Geometry check sheet. Reference: the model listing, model coordinates, mm. Face numbers are marked on the shaded views. A direction names the side the tool comes from. Give positions to 0.01 mm unless a question says otherwise; leave off trailing zeros. Write each loop counter-clockwise with the first axis right and the second up, starting at its lowest first coordinate (ties: lowest second). Pieces come first, ordered by that corner, then holes.
(1) Depth check by flat-ended pin: P1, Ø5, axis at x = 9.5, y = 9.5, coming from the -Z side; P2, Ø1, axis at y = 14, z = 0, coming from the -X side; P3, Ø1, axis at x = 17.5, z = -2.5, coming from the +Y side. Enter the tip coordinate at first touch or a pass-through.
(2) Cross-section at A-A (z = -4). Record the boundary of the cut face in (x, y), and give its area (3 significant figures).
(3) Thickness scan on line 1 along X through (y, z) = (4.25, -7.5); line 2 along Z through (x, y) = (16, 19.5); line 3 along X through (y, z) = (5.5, 2.75). Record the ranges inside material, lowest first.
(4) Tool access check on the marked faces 5, 6, 7, 8 and 9. Record the directions out of +Z, -Z, +X, -X, +Y, -Y that give a thin tool (end or side, any length) a straight path to the whole face; none if there is none.
(5) Cross-section at D-D (y = 10.5). Record the boundary of the cut face in (x, z), and give its area (3 significant figures).
(6) Cross-section at B-B (x = 3.6). Record the boundary of the cut face in (y, z), and give its area (3 significant figures).
(7) Mould release check, pull along Y, two halves, no side actions. Record for the marked faces 1, 2, 3 and 4: +Y half, -Y half, draft (parallel to the pull), parting line (faces both ways), or undercut.
(8) Cross-section at C-C (z = -7). Record the boundary of the cut face in (x, y), and give its area (3 significant figures).
```python
from build123d import *

# Parameters (mm, degrees)
ESQUISSE1_W             = 16.2
ESQUISSE1_H             = 25
BOSS_EXTRU_1_DEPTH      = 3
ESQUISSE2_W             = 13
ESQUISSE2_H             = 8
BOSS_EXTRU_2_DEPTH      = 2
ESQUISSE3_R             = 1.8
BOSS_EXTRU_3_DEPTH      = 1.5
ESQUISSE5_W             = 13
ESQUISSE5_H             = 8
BOSS_EXTRU_4_DEPTH      = 2
ESQUISSE6_R             = 1.8
BOSS_EXTRU_5_DEPTH      = 1.5
ENL_V_MAT_EXTRU_1_REACH = 34.5
ESQUISSE7_W             = 8
ESQUISSE7_H             = 8
ENL_V_MAT_EXTRU_2_REACH = 34.5
ESQUISSE8_R             = 1.75
CONG_1_R                = 1
CONG_2_R                = 4
CONG_3_R                = 2
CONG_4_R                = 2


with BuildPart() as part:
    # Esquisse1 → Boss.-Extru.1 (new body)
    with BuildSketch(Plane.XY):
        with Locations((8.1, 12.5)):
            Rectangle(ESQUISSE1_W, ESQUISSE1_H)
    extrude(amount=BOSS_EXTRU_1_DEPTH)

    # Esquisse2 → Boss.-Extru.2 (add)
    with BuildSketch(Plane.ZY):
        with Locations((-3.5, 4)):
            Rectangle(ESQUISSE2_W, ESQUISSE2_H)
    extrude(amount=BOSS_EXTRU_2_DEPTH)

    # Esquisse3 → Boss.-Extru.3 (add)
    with BuildSketch(Plane(origin=(0, 0, 0), x_dir=(0, 0, -1), z_dir=(1, 0, 0))):
        with Locations(Location((7, 4.035774971, 0), (0, 0, 180))):
            Circle(ESQUISSE3_R)
    extrude(amount=BOSS_EXTRU_3_DEPTH)

    # Esquisse5 → Boss.-Extru.4 (add)
    with BuildSketch(Plane(origin=(16.2, 0, 0), x_dir=(0, 0, -1), z_dir=(1, 0, 0))):
        with Locations((3.5, 4)):
            Rectangle(ESQUISSE5_W, ESQUISSE5_H)
    extrude(amount=BOSS_EXTRU_4_DEPTH)

    # Esquisse6 → Boss.-Extru.5 (add)
    with BuildSketch(Plane.ZY.offset(-16.2)):
        with Locations((-7, 3.879731229)):
            Circle(ESQUISSE6_R)
    extrude(amount=BOSS_EXTRU_5_DEPTH)

    # Esquisse7 → Enlèv. mat.-Extru.1 (cut, up to next)
    with BuildSketch(Plane(origin=(0, 0, 0), x_dir=(-1, 0, 0), z_dir=(0, 0, -1)), mode=Mode.PRIVATE) as enl_v_mat_extru_1_sk1:
        with Locations((-8.1, 4)):
            Rectangle(ESQUISSE7_W, ESQUISSE7_H)
    enl_v_mat_extru_1_tool1 = extrude(enl_v_mat_extru_1_sk1.sketch, amount=-ENL_V_MAT_EXTRU_1_REACH, mode=Mode.PRIVATE) & part.part
    add(enl_v_mat_extru_1_tool1.solids().sort_by_distance((8.1, 4, 0))[0], mode=Mode.SUBTRACT)

    # Esquisse8 → Enlèv. mat.-Extru.2 (cut, up to next)
    with BuildSketch(Plane(origin=(0, 0, 0), x_dir=(-1, 0, 0), z_dir=(0, 0, -1)), mode=Mode.PRIVATE) as enl_v_mat_extru_2_sk1:
        with Locations((-12.6, 18.360124913)):
            Circle(ESQUISSE8_R)
    enl_v_mat_extru_2_tool1 = extrude(enl_v_mat_extru_2_sk1.sketch, amount=-ENL_V_MAT_EXTRU_2_REACH, mode=Mode.PRIVATE) & part.part
    # Esquisse8 → Enlèv. mat.-Extru.2 (cut, up to next)
    with BuildSketch(Plane(origin=(0, 0, 0), x_dir=(-1, 0, 0), z_dir=(0, 0, -1)), mode=Mode.PRIVATE) as enl_v_mat_extru_2_sk2:
        with Locations((-3.6, 18.360124913)):
            Circle(ESQUISSE8_R)
    enl_v_mat_extru_2_tool2 = extrude(enl_v_mat_extru_2_sk2.sketch, amount=-ENL_V_MAT_EXTRU_2_REACH, mode=Mode.PRIVATE) & part.part
    add(enl_v_mat_extru_2_tool1.solids().sort_by_distance((12.6, 18.360125, 0))[0], mode=Mode.SUBTRACT)
    add(enl_v_mat_extru_2_tool2.solids().sort_by_distance((3.6, 18.360125, 0))[0], mode=Mode.SUBTRACT)

    # Congé1
    cong_1_edges = [part.edges().sort_by_distance(p)[0] for p in [
        (14.35, 18.360124913, 0),
        (5.35, 18.360124913, 0),
    ]]
    fillet(cong_1_edges, radius=CONG_1_R)

    # Congé2
    cong_2_edges = [part.edges().sort_by_distance(p)[0] for p in [
        (-1, 8, -10),
        (-1, 0, -10),
        (17.2, 0, -10),
        (17.2, 8, -10),
    ]]
    fillet(cong_2_edges, radius=CONG_2_R - 0.0001)  # a hair under: the kernel refuses the full size

    # Congé3
    cong_3_edges = [part.edges().sort_by_distance(p)[0] for p in [
        (12.1, 0, 1.5),
        (12.1, 8, 1.5),
        (4.1, 8, 1.5),
        (4.1, 0, 1.5),
    ]]
    fillet(cong_3_edges, radius=CONG_3_R)

    # Congé4
    cong_4_edges = [part.edges().sort_by_distance(p)[0] for p in [
        (0, 25, 1.5),
        (16.2, 25, 1.5),
    ]]
    fillet(cong_4_edges, radius=CONG_4_R)


solid = part.part
```
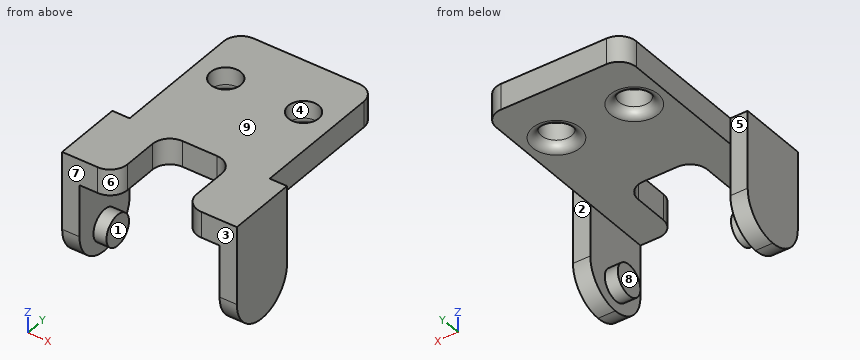
Reply:
1. P1: stops at z = 0
1. P2: stops at x = 0
1. P3: stops at y = 8
2. outline: (-2, 0) - (0, 0) - (0, 8) - (-2, 8) - close; (16.2, 0) - (18.2, 0) - (18.2, 8) - (16.2, 8) - close
2. area: 32.0 mm2
3. line 1: x = -2 to 1.5, 14.7 to 18.2
3. line 2: z = 0 to 3
3. line 3: x = -2 to 4.1, 12.1 to 18.2
4. face 5: +Z, -Z, -X, +Y
4. face 6: +Z, -Z, -Y
4. face 7: +Z, -Z, +X, -X, -Y
4. face 8: -Z, +Y, -Y
4. face 9: +Z, +X, -X, +Y, -Y
5. outline: (0, 0) - (16.2, 0) - (16.2, 3) - (0, 3) - close
5. area: 48.6 mm2
6. outline: (0.68, 0) - (15.61, 0) arc R1 ccw to (16.61, 1) - (16.61, 3) - (0.68, 3) - close; (20.11, 1) arc R1 ccw to (21.11, 0) - (25, 0) - (25, 3) - (20.11, 3) - close
6. area: 62.0 mm2
7. face 1: draft
7. face 2: +Y half
7. face 3: -Y half
7. face 4: undercut
8. outline: (-2, 0.13) - (0, 0.13) - (0, 2.24) - (1.5, 2.24) - (1.5, 5.84) - (0, 5.84) - (0, 7.87) - (-2, 7.87) - close; (14.7, 2.08) - (16.2, 2.08) - (16.2, 0.13) - (18.2, 0.13) - (18.2, 7.87) - (16.2, 7.87) - (16.2, 5.68) - (14.7, 5.68) - close
8. area: 41.8 mm2
